```python
from build123d import *

# Parameters (mm, degrees)
F0_R     = 39.6875
F0_R_2   = 19.84375
F1_DEPTH = 3.175
F0_R_3   = 34.925
F2_DEPTH = 12.7
F3_R     = 4.7625
F5_D     = 12.7


with BuildPart() as f1:
    # F0 (on Front) → F1 (new body, symmetric)
    with BuildSketch(Plane.XZ):
        with BuildLine():
            Line((215.9, -69.85), (215.9, 69.85))
            Line((215.9, 69.85), (-152.4, 69.85))
            ThreePointArc((-152.4, 69.85), (-212.725, 0), (-152.4, -69.85))
            Line((-152.4, -69.85), (215.9, -69.85))
        make_face()
        with Locations((-152.4, 0)):
            Circle(F0_R, mode=Mode.SUBTRACT)
        with Locations((152.4, 0)):
            Circle(F0_R_2, mode=Mode.SUBTRACT)
    extrude(amount=F1_DEPTH, both=True)

    # F0 (on Front) → F2 (join, symmetric)
    with BuildSketch(Plane.XZ):
        with Locations((-152.4, 0)):
            Circle(F0_R)
        with Locations((-152.4, 0)):
            Circle(F0_R_3, mode=Mode.SUBTRACT)
    extrude(amount=F2_DEPTH, both=True)

    # F3
    f3_edges = [f1.edges().sort_by_distance(p)[0] for p in [
        (-192.0875, -3.175, 0),
        (-192.0875, 3.175, 0),
    ]]
    fillet(f3_edges, radius=F3_R)

    # F5 (through all)
    with Locations(Plane(origin=(0, 3.175, 0), x_dir=(-1, 0, 0), z_dir=(0, 1, 0))):
        with Locations((-106.376187, 46.023813), (-198.423813, -46.023813)):
            Hole(F5_D / 2)


solid = f1.part
```
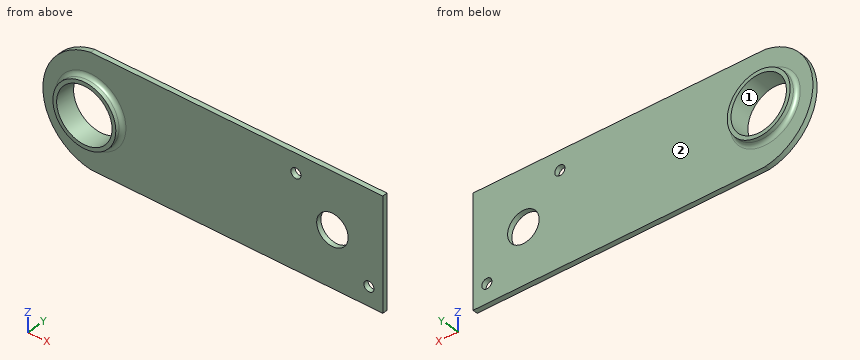
Build history of the part. All positions in model axes, mm. Face numbers are marked on the shaded views. Round coordinates to 2 decimals unless told otherwise and drop trailing zeros. Loops run counter-clockwise (first coordinate to the right, second up) from the corner with the lowest first, then second, coordinate; pieces in that order, holes last.
Item 1: Two-plate mould, pull along Z, no slides. Class the marked faces 1 and 2: released by +Z, released by -Z, zero draft, split by the parting line, or undercut.
Item 2: Saw through at B-B (x = 152.4). List the corners of the cut face in (y, z) (3 decimals), then the cut area to 3 significant figures.
Item 3: Pin check, flat tips, straight feed: P1, Ø1, axis at x = 170, z = 42.5, coming from the -Y side (3 decimals); P2, Ø8, axis at x = -117.5, z = 29, coming from the -Y side; P3, Ø12, axis at x = 27, z = 22.5, coming from the +Y side (3 decimals). Stop position of each tip, or through.
Item 4: Drill centre lines: line 1 along Z through (x, y) = (152.4, 1.5); line 2 along Y through (x, z) = (162.5, -54) (3 decimals); line 3 along Z through (x, y) = (-121, 9.75). Where is each one in solid material? Low to high.
Item 5: Saw through at A-A (z = 0). State how many separate pieces and enclosed holes the cut face has, then the cut area to 3 significant figures.
Worked answers:
1. face 1: undercut
1. face 2: zero draft
2. outline: (-3.175, -69.85) - (3.175, -69.85) - (3.175, -19.844) - (-3.175, -19.844) - close; (-3.175, 19.844) - (3.175, 19.844) - (3.175, 69.85) - (-3.175, 69.85) - close
2. area: 635 mm2
3. P1: stops at y = -3.175
3. P2: stops at y = -4.3
3. P3: stops at y = 3.175
4. line 1: z = -69.85 to -19.84, 19.84 to 69.85
4. line 2: y = -3.175 to 3.175
4. line 3: z = -24.27 to -15.29, 15.29 to 24.27
5. separate pieces: 3
5. enclosed holes: 0
5. area: 2,230 mm2
